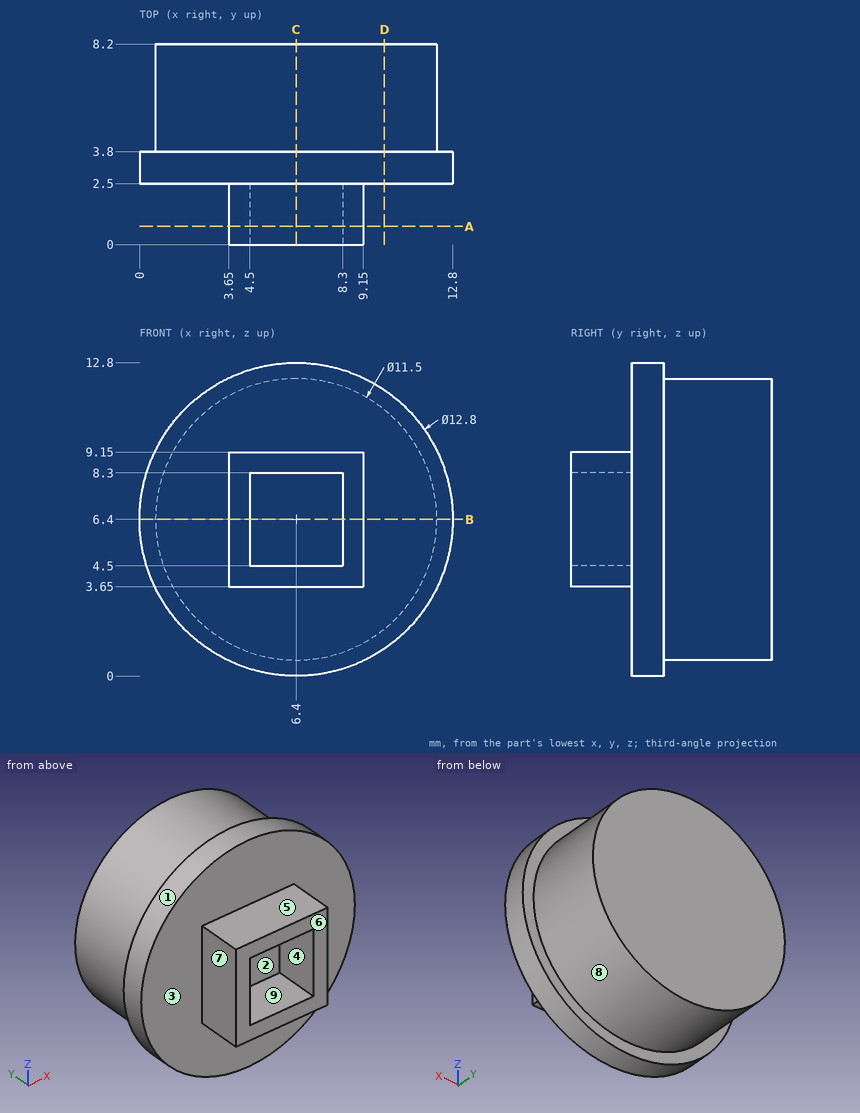
Verification items for this drawing (mm, ordinates from the low corner). A direction names the side the tool comes from. Coordinates: 2 decimals unless noted, no trailing zeros. Write each loop counter-clockwise with the first axis right and the second up, starting at its lowest first coordinate (ties: lowest second). Pieces come first, ordered by that corner, then holes. Notation, with made-up numbers: M 51.5,-7.5 L 105.5,-7.5 A18 ccw 105.5,25.5 Z; hole C 79,40.25 d5. An arc over 180 degrees is marked long. Answer as CSV lines item,"result".
Q1. Material ranges on probe 1 along Z at (x, y) = (6, 1.5); probe 2 along Y at (x, z) = (3.25, 2.75), recorded low to high. Write a range as from..to.
Check result:
probe 1,"3.65..4.5, 8.3..9.15"
probe 2,"2.5..8.2"
Q2. Cross-section at A-A (y = 0.75). Record the boundary of the cut face in (x, z).
Check result:
outline,"M 3.65,3.65 L 9.15,3.65 L 9.15,9.15 L 3.65,9.15 Z; hole M 4.5,4.5 L 8.3,4.5 L 8.3,8.3 L 4.5,8.3 Z"
Q3. Mould release check, pull along X, two halves, no side actions. Record for the marked faces 1, 2, 3 and 4: released by +X, released by -X, zero draft, split by the parting line, or undercut.
Check result:
face 1,"split by the parting line"
face 2,"undercut"
face 3,"zero draft"
face 4,"undercut"
Q4. Go/stop test with flat-tipped pins: pin 1 (1.5 mm diameter, centred on x = 4.5, y = 5.5, fed in from +Z); pin 2 (0.8 mm diameter, centred on x = 5.5, y = 2, fed in from +Z); pin 3 (0.8 mm diameter, centred on x = 7, y = 1.5, fed in from -Z). Record where each tip stops, or that it passes through.
Check result:
pin 1,"z = 12.03"
pin 2,"z = 9.15"
pin 3,"z = 3.65"
Q5. Cross-section at C-C (x = 6.4). Record the boundary of the cut face in (y, z), then the cut area to 3 significant figures.
Check result:
outline,"M 0,3.65 L 2.5,3.65 L 2.5,0 L 3.8,0 L 3.8,0.65 L 8.2,0.65 L 8.2,12.15 L 3.8,12.15 L 3.8,12.8 L 2.5,12.8 L 2.5,9.15 L 0,9.15 L 0,8.3 L 2.5,8.3 L 2.5,4.5 L 0,4.5 Z"
area,"71.5 mm^2"
Q6. Set-up check for the marked faces 5, 6, 7, 8 and 9: record each of +Z, -Z, +X, -X, +Y, -Y from which the full face is reachable in a straight line by a thin tool's end or side.
Check result:
face 5,"+Z, +X, -X, -Y"
face 6,"+Z, -Z, +X, -X, -Y"
face 7,"+Z, -Z, -X, -Y"
face 8,"+Y"
face 9,"-Y"
Q7. Cross-section at D-D (x = 10). Record the boundary of the cut face in (y, z), then the cut area to 3 significant figures.
Check result:
outline,"M 2.5,1.11 L 3.8,1.11 L 3.8,1.92 L 8.2,1.92 L 8.2,10.88 L 3.8,10.88 L 3.8,11.69 L 2.5,11.69 Z"
area,"53.2 mm^2"
Q8. Cross-section at B-B (z = 6.4). Record the boundary of the cut face in (x, y).
Check result:
outline,"M 0,2.5 L 3.65,2.5 L 3.65,0 L 4.5,0 L 4.5,2.5 L 8.3,2.5 L 8.3,0 L 9.15,0 L 9.15,2.5 L 12.8,2.5 L 12.8,3.8 L 12.15,3.8 L 12.15,8.2 L 0.65,8.2 L 0.65,3.8 L 0,3.8 Z"
